from build123d import *

# Parameters (mm, degrees)
F0_W     = 104.791857
F0_H     = 60.042905
F1_DEPTH = 66.548
F3_W     = 87.298889
F3_H     = 39.771117
F4_DEPTH = 60.043905
F2_W     = 35.969097
F2_H     = 22.374479
F5_DEPTH = 66.549
F6_R     = 6.173541
F7_DEPTH = 104.792857


with BuildPart() as f1:
    # F0 (on Front) → F1 (new body)
    with BuildSketch(Plane.XZ):
        with Locations((2.407379, -0.566443)):
            Rectangle(F0_W, F0_H)
    extrude(amount=F1_DEPTH)

    # F3 (on face) → F4 (cut, through all)
    with BuildSketch(Plane.XY.offset(29.45501)):
        with Locations((0.584687, -31.723138)):
            Rectangle(F3_W, F3_H)
    extrude(amount=-F4_DEPTH, mode=Mode.SUBTRACT)

    # F2 (on face) → F5 (cut, through all)
    with BuildSketch(Plane.XZ.offset(66.548)):
        with Locations((0.849664, 18.26777)):
            Rectangle(F2_W, F2_H)
    extrude(amount=-F5_DEPTH, mode=Mode.SUBTRACT)

    # F6 (on face) → F7 (cut, through all)
    with BuildSketch(Plane.YZ.offset(54.803308)):
        with Locations((-32.995041, -0.901195)):
            Circle(F6_R)
    extrude(amount=-F7_DEPTH, mode=Mode.SUBTRACT)


solid = f1.part
Work out the finished part from the listing and answer in its coordinate system (mm). A direction names the side the tool comes from. Round coordinates to 2 decimals unless told otherwise and drop trailing zeros. Write each loop counter-clockwise with the first axis right and the second up, starting at its lowest first coordinate (ties: lowest second). Pieces come first, ordered by that corner, then holes. Notation, with made-up numbers: (46.5, 9.5) - (80.5, 9.5) arc R19 ccw to (80.5, 31.5) - close; hole circle Ø5 at (72.25, 80). An arc over 180 degrees is marked (long way). Answer in a Markdown table with one row per item. Add a question column.
1. Find the intervals of material crossed by line 1 along X through (y, z) = (-48.5, -9.5); line 2 along Y through (x, z) = (3.5, -7); line 3 along X through (y, z) = (-8.5, 21), in increasing order. Write a range as from..to.
2. A cutting plane is placed at B-B, the plane z = 17.5. Determine the outline of the cut face in (x, y).
3. A cutting plane is placed at C-C, the plane x = -3. Determine the outline of the cut face in (y, z).
4. The mould has two halves that part along X. Classify faces 4 (the flat face through (0, -51.609, 0)), 5 (the flat face through (-49.989, -33, -8)), 6 (the flat face through (45, -33, 29.455)), 7 (the flat face through (1, -6, 7.081)): +X half, -X half, draft (parallel to the pull), parting line (faces both ways), or undercut.
5. A cutting plane is placed at A-A, the plane y = -42.5. Determine the outline of the cut face in (x, z) (3 decimals).
6. For faces 1 (the flat face through (2, -66.548, 0)), 2 (the flat face through (18.834, -59, 18)), 3 (the flat face through (44.234, -32, 7)), determine the directions among +Z, -Z, +X, -X, +Y, -Y from which every point of the face is accessible in a straight line to the end or side of a thin tool.
7. A cutting plane is placed at D-D, the plane z = -21.5. Determine the outline of the cut face in (x, y), and give its area (3 significant figures).
8. Given pin 1 (18 mm diameter, centred on x = 17, z = 10, fed in from -Y); pin 2 (7.5 mm diameter, centred on x = 1.5, y = -60.5, fed in from +Z); pin 3 (11 mm diameter, centred on y = -33, z = -0.9, fed in from +X), each flat-ended and moving along its own axis, determine where each tip first touches the part or whether it passes through.
Worked out:
| question | item | result |
|---|---|---|
| 1 | line 1 | -49.99..-43.06, 44.23..54.8 |
| 1 | line 2 | -66.55..-51.61, -11.84..0 |
| 1 | line 3 | -49.99..-17.13, 18.83..54.8 |
| 2 | outline | (-49.99, -66.55) - (-17.13, -66.55) - (-17.13, -51.61) - (-43.06, -51.61) - (-43.06, -11.84) - (-17.13, -11.84) - (-17.13, 0) - (-49.99, 0) - close; (18.83, -66.55) - (54.8, -66.55) - (54.8, 0) - (18.83, 0) - (18.83, -11.84) - (44.23, -11.84) - (44.23, -51.61) - (18.83, -51.61) - close |
| 3 | outline | (-66.55, -30.59) - (-51.61, -30.59) - (-51.61, 7.08) - (-66.55, 7.08) - close; (-11.84, -30.59) - (0, -30.59) - (0, 7.08) - (-11.84, 7.08) - close |
| 4 | face 4 | undercut |
| 4 | face 5 | -X half |
| 4 | face 6 | draft |
| 4 | face 7 | undercut |
| 5 | outline | (-49.989, -30.588) - (-43.065, -30.588) - (-43.065, 29.455) - (-49.989, 29.455) - close; (44.234, -30.588) - (54.803, -30.588) - (54.803, 29.455) - (44.234, 29.455) - close |
| 6 | face 1 | +Z, -Z, +X, -X, -Y |
| 6 | face 2 | +Z, +Y, -Y |
| 6 | face 3 | +Z, -Z |
| 7 | outline | (-49.99, -66.55) - (54.8, -66.55) - (54.8, 0) - (-49.99, 0) - close; hole (-43.06, -51.61) - (44.23, -51.61) - (44.23, -11.84) - (-43.06, -11.84) - close |
| 7 | area | 3,500 mm^2 |
| 8 | pin 1 | y = -66.55 |
| 8 | pin 2 | z = 7.08 |
| 8 | pin 3 | through |
